from build123d import *

# Parameters (mm, degrees)
F0_W     = 12
F0_H     = 12
F1_DEPTH = 12
F3_START = 3
F2_W     = 6
F2_H     = 6
F3_DEPTH = 6


with BuildPart() as f1:
    # F0 (on Top) → F1 (new body)
    with BuildSketch(Plane.XY):
        with Locations((-6, -6)):
            Rectangle(F0_W, F0_H)
    extrude(amount=F1_DEPTH)

    # F2 (on Top) → F3 (cut)
    with BuildSketch(Plane.XY.offset(F3_START)):
        with Locations((-6, -6)):
            Rectangle(F2_W, F2_H)
    extrude(amount=F3_DEPTH, mode=Mode.SUBTRACT)


solid = f1.part
The model under review builds one solid part; all positions refer to its coordinate system, in mm. A direction names the side the tool comes from. Give positions to 0.01 mm unless a question says otherwise; leave off trailing zeros. Loops run counter-clockwise (first coordinate to the right, second up) from the corner with the lowest first, then second, coordinate; pieces in that order, holes last. Notation, with made-up numbers: (18.25, 19.5) -> (49.25, 19.5) arc R12 cw to (49.25, 29.5) -> close; hole circle Ø7 at (-39, -8). An arc over 180 degrees is marked (long way). Put each result on its own line as item: value. Start each with the question number.
1. We need section B-B on x = -3.5. State the section outline as (y, z) points, then the cut area to 3 significant figures.
2. We need section A-A on z = 8.75. State the section outline as (x, y) points, then the cut area to 3 significant figures.
3. Mouldability with a two-part tool opening along Z and no side actions: class faces 3 (the face through (-12, -6, 6)), 4 (the face through (-9, -6, 6)), 5 (the face through (-6, -6, 3)), 6 (the face through (-6, -6, 12)) as released by +Z, released by -Z, zero draft, split by the parting line, or undercut.
4. Wall thickness on probe 1 along X at (y, z) = (-6.5, 8.25); probe 2 along Z at (x, y) = (-5.25, -7.75): over which ranges is each line inside the solid? List them lowest first.
5. For faces 1 (the face through (0, -6, 6)), 2 (the face through (-6, -6, 9)), list the 3-axis set-ups (+Z, -Z, +X, -X, +Y, -Y) from which the entire face can be reached by the end or side of a thin tool; tool diameter is ignored.
Determined:
1. outline: (-12, 0) -> (0, 0) -> (0, 12) -> (-12, 12) -> close; hole (-9, 3) -> (-3, 3) -> (-3, 9) -> (-9, 9) -> close
1. area: 108 mm^2
2. outline: (-12, -12) -> (0, -12) -> (0, 0) -> (-12, 0) -> close; hole (-9, -9) -> (-3, -9) -> (-3, -3) -> (-9, -3) -> close
2. area: 108 mm^2
3. face 3: zero draft
3. face 4: undercut
3. face 5: undercut
3. face 6: released by +Z
4. probe 1: -12 to -9, -3 to 0
4. probe 2: 0 to 3, 9 to 12
5. face 1: +Z, -Z, +X, +Y, -Y
5. face 2: none
